Can you work these out from the model? Positions are in its coordinate system, mm. A direction names the side the tool comes from. Coordinates: 2 decimals unless noted, no trailing zeros. Order: outer loops, then holes, each group sorted by start corner. A loop starts at its lowest first (then second) coordinate and runs counter-clockwise, first axis right, second up. Notation, with made-up numbers: (61, 23.25) -> (100, 23.25) arc R10 ccw to (100, 31.25) -> close; hole circle Ø5 at (15, -18.5). An arc over 180 degrees is marked (long way). Answer as a JSON object with one key per item and string values. Group by question number.
(1) I want a section at C-C, the plane z = 4.5. List the corners of the cut face in (x, y) for me.
(2) Which directions (+Z, -Z, +X, -X, +Y, -Y) give clear straight access to the entire face, cutting with the end or side of a thin tool? Please do faces 1 (the flat face through (-2, -1, -30.162)), 2 (the cylindrical face through (-0.43, -1.92, 35.64)), 3 (the cylindrical face through (2.65, 0.83, 0.42)).
(3) I want a section at A-A, the plane x = 0. List the corners of the cut face in (y, z) for me (1 decimal).
(4) For pin 1 (2 mm diameter, centred on x = -2, y = 1, fed in from +Z) (3 decimals); pin 2 (1.5 mm diameter, centred on y = -1.5, z = -30.5, fed in from -X); pin 3 (1 mm diameter, centred on x = 1.5, z = 7, fed in from -Y), each with a flat end and sliding along its axis, tell me the tip position at first contact or that it passes through.
(5) I need wall thicknesses on line 1 (X direction, y = -0.3, z = -20); line 2 (Z direction, x = -1.5, y = 1.65); line 3 (Y direction, x = -0.2, z = -22). Which ranges of each line are inside material? Lowest first, please.
from build123d import *

# Parameters (mm, degrees)
SKETCH2_R      = 2.778125
EXTRUDE1_DEPTH = 30.1625
SKETCH3_R      = 1.9685
EXTRUDE2_DEPTH = 11.1125
SKETCH4_R      = 1.9685
EXTRUDE3_DEPTH = 11.1125


with BuildPart() as part:
    # Sketch2 → Extrude1 (new body, symmetric)
    with BuildSketch(Plane.XY):
        Circle(SKETCH2_R)
    extrude(amount=EXTRUDE1_DEPTH, both=True)

    # Sketch3 → Extrude2 (add)
    with BuildSketch(Plane.XY.offset(30.1625)):
        Circle(SKETCH3_R)
    extrude(amount=EXTRUDE2_DEPTH)

    # Sketch4 → Extrude3 (add)
    with BuildSketch(Plane(origin=(0, 0, -30.1625), x_dir=(-1, 0, 0), z_dir=(0, 0, -1))):
        Circle(SKETCH4_R)
    extrude(amount=EXTRUDE3_DEPTH)


solid = part.part
Computed values:
{
 "1": {"outline": "circle Ø5.56 at (0, 0)"},
 "2": {"face 1": "-Z", "face 2": "+Z", "face 3": "+Z, -Z"},
 "3": {"outline": "(-2.8, -30.2) -> (-2, -30.2) -> (-2, -41.3) -> (2, -41.3) -> (2, -30.2) -> (2.8, -30.2) -> (2.8, 30.2) -> (2, 30.2) -> (2, 41.3) -> (-2, 41.3) -> (-2, 30.2) -> (-2.8, 30.2) -> close"},
 "4": {"pin 1": "stops at z = 41.275", "pin 2": "stops at x = -2.65", "pin 3": "stops at y = -2.59"},
 "5": {"line 1": "x = -2.76 to 2.76", "line 2": "z = -30.16 to 30.16", "line 3": "y = -2.77 to 2.77"}
}
